from build123d import *

# Parameters (mm, degrees)
SKETCH1_W           = 121
SKETCH1_H           = 13
BOSS_EXTRUDE1_DEPTH = 28.5
SKETCH2_R           = 6.5
CUT_EXTRUDE1_DEPTH  = 69.128554953
BOSS_EXTRUDE2_DEPTH = 57
CUT_EXTRUDE3_REACH  = 93.09
CUT_EXTRUDE4_REACH  = 93.09


with BuildPart() as part:
    # Sketch1 → Boss-Extrude1 (new, symmetric)
    with BuildSketch(Plane.XY):
        with Locations((0, 6.5)):
            Rectangle(SKETCH1_W, SKETCH1_H)
    extrude(amount=BOSS_EXTRUDE1_DEPTH, both=True)

    # Sketch2 → Cut-Extrude1 (cut, through all)
    with BuildSketch(Plane(origin=(0, 13, 0), x_dir=(1, 0, 0), z_dir=(0, 1, 0))):
        with Locations(Location((-44.5, 12.5, 0), (0, 0, 270))):
            Circle(SKETCH2_R)
        with Locations(Location((-44.5, -12.5, 0), (0, 0, 270))):
            Circle(SKETCH2_R)
    extrude(amount=-CUT_EXTRUDE1_DEPTH, mode=Mode.SUBTRACT)

    # Sketch3 → Boss-Extrude2 (add)
    with BuildSketch(Plane.XY.offset(28.5)):
        Polygon((-25.5, 13), (-25.5, 54), (33.5, 38.190997647), (60.5, 22.602540378), (60.5, 13), align=None)
    extrude(amount=-BOSS_EXTRUDE2_DEPTH)

    # Sketch7 → Cut-Extrude3 (cut, up to next)
    with BuildSketch(Plane(origin=(6.940887603, 25.903745183, 25.903745183), x_dir=(0.9825200508486979, -0.13163272708614732, -0.13163272708614732), z_dir=(0.1861567878973858, 0.6947465906068656, 0.6947465906068659)), mode=Mode.PRIVATE) as cut_extrude3_sk1:
        Polygon((-40.951405202, -0.627191909), (-40.951405202, 40.505985035), (61.941772905, 20.980207657), (61.941772905, -20.152969287), align=None)
    cut_extrude3_tool1 = extrude(cut_extrude3_sk1.sketch, amount=CUT_EXTRUDE3_REACH, mode=Mode.PRIVATE) & part.part
    add(cut_extrude3_tool1.solids().sort_by_distance((17.252616, 31.718113, 17.326358))[0], mode=Mode.SUBTRACT)

    # Sketch10 → Cut-Extrude4 (cut, up to next)
    with BuildSketch(Plane(origin=(6.940887603, 25.903745183, -25.903745183), x_dir=(-0.9825200508486979, 0.13163272708614734, -0.13163272708614734), z_dir=(0.18615678789738585, 0.6947465906068656, -0.6947465906068659)), mode=Mode.PRIVATE) as cut_extrude4_sk1:
        Polygon((44.988619568, 4.703278136), (44.988619568, 35.815976509), (-66.918136798, 14.9837742), (-66.918136798, -16.128924173), align=None)
    cut_extrude4_tool1 = extrude(cut_extrude4_sk1.sketch, amount=CUT_EXTRUDE4_REACH, mode=Mode.PRIVATE) & part.part
    add(cut_extrude4_tool1.solids().sort_by_distance((17.713983, 31.420848, -17.5))[0], mode=Mode.SUBTRACT)


solid = part.part
Input: part model. Units: mm. Frame: model coordinates. A direction names the side the tool comes from. Give positions to 0.01 mm unless a question says otherwise; leave off trailing zeros. Order: outer loops, then holes, each group sorted by start corner. A loop starts at its lowest first (then second) coordinate and runs counter-clockwise, first axis right, second up.
Q1. Section C-C on x = -21. Output: boundary loops of the cut face in (y, z).
Checked values:
outline: (0, -28.5) - (30.79, -28.5) - (52.79, -6.5) - (52.79, 6.5) - (30.79, 28.5) - (0, 28.5) - close
Q2. Section D-D on y = 48. Output: boundary loops of the cut face in (x, z), and give its area (3 significant figures).
Checked values:
outline: (-25.5, -12.5) - (-3.11, -6.5) - (-3.11, 6.5) - (-25.5, 12.5) - close
area: 425 mm2
Q3. Draft query along Y for faces 3 (the flat face through (18.102, 31.632, 17.185)), 4 (the flat face through (-1, 0, 0)), 5 (the flat face through (60.5, 11, 0)). Return one class per face: +Y half, -Y half, draft (parallel to the pull), parting line (faces both ways), or undercut.
Checked values:
face 3: +Y half
face 4: -Y half
face 5: draft
Q4. Section A-A on x = -44.5. Output: boundary loops of the cut face in (y, z).
Checked values:
outline: (0, -28.5) - (13, -28.5) - (13, -19) - (0, -19) - close; (0, -6) - (13, -6) - (13, 6) - (0, 6) - close; (0, 19) - (13, 19) - (13, 28.5) - (0, 28.5) - close
Q5. Contact query for flat-ended pins moving along their axis: pin 1 Ø8 at (x, z) = (-5.5, 2) entering from +Y; pin 2 Ø3 at (x, y) = (-15, 38) entering from +Z; pin 3 Ø5 at (x, z) = (2.5, -7) entering from +Y; pin 4 Ø11.5 at (x, z) = (-44.5, -12.5) entering from -Y. Output: stop coordinate, or through.
Checked values:
pin 1: stops at y = 49.71
pin 2: stops at z = 21.24
pin 3: stops at y = 47.15
pin 4: passes through
Q6. Set-up query: faces 1 (the flat face through (-25.5, 29, 0)), 2 (the flat face through (49.811, 28.774, 0.208)). Return all of +Z, -Z, +X, -X, +Y, -Y with unobstructed straight access to the full face (end or side cutting, diameter ignored); none if empty.
Checked values:
face 1: +Z, -Z, -X, +Y
face 2: +Z, -Z, +X, +Y
Q7. Section B-B on z = -12.5. Output: boundary loops of the cut face in (x, y).
Checked values:
outline: (-60.5, 0) - (-51, 0) - (-51, 13) - (-60.5, 13) - close; (-38, 0) - (60.5, 0) - (60.5, 22.6) - (52.89, 26.99) - (-25.5, 48) - (-25.5, 13) - (-38, 13) - close
Q8. Ray query, probe 1 along Z at (x, y) = (-44, 3); probe 2 along X at (y, z) = (8, 12.5); probe 3 along Y at (x, z) = (-53.5, -16.5). Return the intervals inside material, ascending.
Checked values:
probe 1: z = -28.5 to -18.98, -6.02 to 6.02, 18.98 to 28.5
probe 2: x = -60.5 to -51, -38 to 60.5
probe 3: y = 0 to 13
